from build123d import *

# Parameters (mm, degrees)
SKETCH1_W           = 25.4
SKETCH1_H           = 25.4
BOSS_EXTRUDE1_DEPTH = 222.25
SKETCH2_W           = 2.54
SKETCH2_H           = 82.55
CUT_EXTRUDE1_DEPTH  = 222.25
SKETCH3_R           = 6.35
SKETCH3_R_2         = 3.175
CUT_EXTRUDE2_DEPTH  = 222.25
SKETCH4_W           = 76.2
SKETCH4_H           = 101.6
BOSS_EXTRUDE3_DEPTH = 6.35


with BuildPart() as part:
    # Sketch1 → Boss-Extrude1 (new body)
    with BuildSketch(Plane(origin=(0, 0, 0), x_dir=(1, 0, 0), z_dir=(0, 1, 0))):
        Rectangle(SKETCH1_W, SKETCH1_H)
    extrude(amount=BOSS_EXTRUDE1_DEPTH)

    # Sketch2 → Cut-Extrude1 (cut)
    with BuildSketch(Plane.XY.offset(12.7)):
        with Locations((-11.43, 41.275)):
            Rectangle(SKETCH2_W, SKETCH2_H)
        with Locations((11.43, 41.275)):
            Rectangle(SKETCH2_W, SKETCH2_H)
    extrude(amount=-CUT_EXTRUDE1_DEPTH, mode=Mode.SUBTRACT)

    # Sketch3 → Cut-Extrude2 (cut)
    with BuildSketch(Plane(origin=(12.7, 0, 0), x_dir=(0, 0, -1), z_dir=(1, 0, 0))):
        with Locations((0, 209.55)):
            Circle(SKETCH3_R)
        with Locations(Location((6.35, 69.85, 0), (0, 0, 90))):
            Circle(SKETCH3_R_2)
        with Locations(Location((6.35, 29.21, 0), (0, 0, 90))):
            Circle(SKETCH3_R_2)
    extrude(amount=-CUT_EXTRUDE2_DEPTH, mode=Mode.SUBTRACT)

    # Sketch4 → Boss-Extrude3 (add)
    with BuildSketch(Plane.XY.offset(12.7)):
        with Locations((0, 50.8)):
            Rectangle(SKETCH4_W, SKETCH4_H)
    extrude(amount=BOSS_EXTRUDE3_DEPTH)


solid = part.part
Work out the finished part from the listing and answer in its coordinate system (mm). A direction names the side the tool comes from. Give positions to 0.01 mm unless a question says otherwise; leave off trailing zeros. Order: outer loops, then holes, each group sorted by start corner. A loop starts at its lowest first (then second) coordinate and runs counter-clockwise, first axis right, second up. Notation, with made-up numbers: M -17,-36.5 L 21,-36.5 A9 ccw 21,-24.5 Z; hole C 82.5,36 d10. An arc over 180 degrees is marked long. Return JSON: item names as keys, results as strings.
Q1. Find section B-B, the plane z = 3. Write down the section's boundary in (x, y), and give its area (3 significant figures).
Answer below:
{"outline": "M -12.7,82.55 L -10.16,82.55 L -10.16,0 L 10.16,0 L 10.16,82.55 L 12.7,82.55 L 12.7,203.95 L -12.7,203.95 Z; M -12.7,215.15 L 12.7,215.15 L 12.7,222.25 L -12.7,222.25 Z", "area": "4,940 mm^2"}
Q2. Each of these flat-tipped pins is pushed along its axis until it touches: pin 1 (6 mm diameter, centred on y = 131, z = 10.5, fed in from +X); pin 2 (12.5 mm diameter, centred on y = 23, z = 5, fed in from -X); pin 3 (4 mm diameter, centred on y = 69.85, z = -6.35, fed in from +X); pin 4 (7.5 mm diameter, centred on y = 185.5, z = 3.5, fed in from -X). Where does it stop, or does it pass through?
Answer below:
{"pin 1": "stops at x = 12.7", "pin 2": "stops at x = -10.16", "pin 3": "passes through", "pin 4": "stops at x = -12.7"}
Q3. Find section A-A, the plane y = 209.55. Write down the section's boundary in (x, z), and give its area (3 significant figures).
Answer below:
{"outline": "M -12.7,-12.7 L 12.7,-12.7 L 12.7,-6.35 L -12.7,-6.35 Z; M -12.7,6.35 L 12.7,6.35 L 12.7,12.7 L -12.7,12.7 Z", "area": "323 mm^2"}
Q4. Find section C-C, the plane x = -6. Write down the section's boundary in (y, z) (3 decimals).
Answer below:
{"outline": "M 0,-12.7 L 222.25,-12.7 L 222.25,12.7 L 101.6,12.7 L 101.6,19.05 L 0,19.05 Z; hole C 29.21,-6.35 d6.35; hole C 69.85,-6.35 d6.35; hole C 209.55,0 d12.7"}
Q5. The mould has two halves that part along Y. Classify faces 6 (the face through (-38.1, 50, 16)), 7 (the face through (0.14, 67.33, -8.28)), 8 (the face through (-1, 101.6, 16)): pulls with the +Y half, pulls with the -Y half, needs draft (parallel to the pull), parting line crosses it, or undercut.
Answer below:
{"face 6": "needs draft", "face 7": "undercut", "face 8": "pulls with the +Y half"}
Q6. Find section D-D, the plane y = 58. Write down the section's boundary in (x, z), and give its area (4 significant figures).
Answer below:
{"outline": "M -38.1,12.7 L -10.16,12.7 L -10.16,-12.7 L 10.16,-12.7 L 10.16,12.7 L 38.1,12.7 L 38.1,19.05 L -38.1,19.05 Z", "area": "1,000 mm^2"}
Q7. Find the intervals of material crossed by line 1 along Z through (x, y) = (-4, 29.21) (3 decimals); line 2 along Y through (x, z) = (-11, 17); line 3 along X through (y, z) = (80, -3), in increasing order. Write a range as [from, to].
Answer below:
{"line 1": "z = [-12.7, -9.525], [-3.175, 19.05]", "line 2": "y = [0, 101.6]", "line 3": "x = [-10.16, 10.16]"}
Q8. Which of the six approach directions +Z, -Z, +X, -X, +Y, -Y give full straight-line access (tool end or side, diameter ignored) to faces 1 (the face through (0.14, 32.14, -7.57)), 2 (the face through (0, 161, 12.7)), 3 (the face through (10.16, 41, 0)), 4 (the face through (38.1, 50, 16)), 5 (the face through (-10.16, 41, 0))?
Answer below:
{"face 1": "+X, -X", "face 2": "+Z, +X, -X, +Y", "face 3": "-Z, +X, -Y", "face 4": "+Z, -Z, +X, +Y, -Y", "face 5": "-Z, -X, -Y"}
